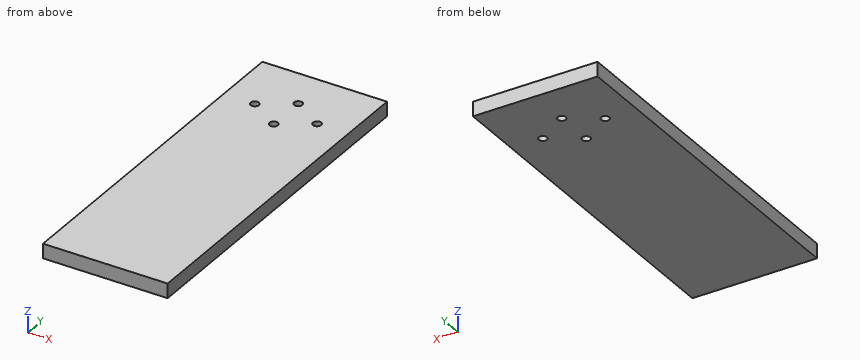
Autodesk Inventor part; units mm, degrees
ref_plane "YZ Plane" through (0, 0, 0) normal (1, 0, 0) x (0, 1, 0)
ref_plane "XZ Plane" through (0, 0, 0) normal (0, 1, 0) x (-1, 0, 0)
ref_plane "XY Plane" through (0, 0, 0) normal (0, 0, 1) x (1, 0, 0)
sketch "Sketch1" plane through (0, 0, 0) normal (0, 0, 1) x (1, 0, 0)
  line L0 (0, 0) -> (-7.5, 0) construction
  line L1 (0, 0) -> (0, 4.75) construction
  line L2 (0, 0) -> (0, 15)
  line L3 (0, 15) -> (-15, 15)
  line L4 (-15, 15) -> (-15, -70)
  line L5 (-15, -70) -> (0, -70)
  line L6 (0, -70) -> (0, 0)
  dimension "d10" = 7.5
  dimension "d14" = 4.75
  dimension "d17" = 15
  dimension "d18" = 15
  dimension "d19" = 70
extrude "Extrusion1" add sketch "Sketch1" along normal blind 3.5
hole "Hole1" at (0, 4.75, 0) at (-7.5, 0, 0) direction (0, 0, 1) diameter 2 end through all
mirror "Mirror2" about plane through (0, 0, 0) normal (0, 1, 0) of "Hole1"
mirror "Mirror1" about plane through (0, 0, 0) normal (1, 0, 0)
properties part number "segment3a" material "Plywood, Finish"
Read the model definition and answer for the solid it produces. Units are mm, in the model's axes. Give positions to 0.01 mm unless a question says otherwise; leave off trailing zeros. Order: outer loops, then holes, each group sorted by start corner. A loop starts at its lowest first (then second) coordinate and runs counter-clockwise, first axis right, second up. Notation, with made-up numbers: (0.25, 47.5) -> (50.25, 47.5) arc R22 cw to (50.25, 77.5) -> close; hole circle Ø5 at (-38.75, -39.5). An arc over 180 degrees is marked (long way). One line per item, written item: value. Start each with the question number.
(1) The part is cut by section C-C (x = 7.5). Determine the outline of the cut face in (y, z).
(2) The part is cut by section B-B (y = 4.75). Determine the outline of the cut face in (x, z), and give its area (3 significant figures).
(3) The part is cut by section A-A (x = 0). Determine the outline of the cut face in (y, z).
(4) Straight lines are drawn through the part: L1, parallel to X at y = 0, z = 1.75; L2, parallel to X at y = 4.75, z = 2.25; L3, parallel to Y at x = 7.5, z = 0.8. For each, find the intervals that lie inside material, in ascending order.
Taken from the geometry:
1. outline: (-70, 0) -> (-1, 0) -> (-1, 3.5) -> (-70, 3.5) -> close; (1, 0) -> (15, 0) -> (15, 3.5) -> (1, 3.5) -> close
2. outline: (-15, 0) -> (-1, 0) -> (-1, 3.5) -> (-15, 3.5) -> close; (1, 0) -> (15, 0) -> (15, 3.5) -> (1, 3.5) -> close
2. area: 98.0 mm^2
3. outline: (-70, 0) -> (-5.75, 0) -> (-5.75, 3.5) -> (-70, 3.5) -> close; (-3.75, 0) -> (3.75, 0) -> (3.75, 3.5) -> (-3.75, 3.5) -> close; (5.75, 0) -> (15, 0) -> (15, 3.5) -> (5.75, 3.5) -> close
4. L1: -15 to -8.5, -6.5 to 6.5, 8.5 to 15
4. L2: -15 to -1, 1 to 15
4. L3: -70 to -1, 1 to 15
